from build123d import *

# Parameters (mm, degrees)
SKETCH1_W           = 20.32
SKETCH1_H           = 50.8
BOSS_EXTRUDE1_DEPTH = 19.05
CUT_EXTRUDE1_DEPTH  = 50.8
SKETCH5_W           = 3.175
SKETCH5_H           = 3.175
CUT_EXTRUDE2_DEPTH  = 50.8


with BuildPart() as part:
    # Sketch1 → Boss-Extrude1 (new body)
    with BuildSketch(Plane(origin=(0, 0, 0), x_dir=(1, 0, 0), z_dir=(0, 1, 0))):
        Rectangle(SKETCH1_W, SKETCH1_H)
    extrude(amount=BOSS_EXTRUDE1_DEPTH)

    # Sketch3 → Cut-Extrude1 (cut)
    with BuildSketch(Plane.XY.offset(25.4)):
        Polygon((-4.233333333, 3.81), (4.233333333, 3.81), (2.116666667, 1.905), (4.233333333, 0), (-4.233333333, 0), (-2.116666667, 1.905), align=None)
    extrude(amount=-CUT_EXTRUDE1_DEPTH, mode=Mode.SUBTRACT)

    # Sketch4 → Revolve1 (revolve)
    with BuildSketch(Plane.XZ.offset(-3.81)):
        with BuildLine():
            Line((0, 4.7413418), (0, 3.4713418))
            ThreePointArc((0, 3.4713418), (0.635, 4.1063418), (0, 4.7413418))
        make_face()
    revolve(axis=Axis((0, 3.81, -25.4), (0, 0, 1)))

    # Sketch5 → Cut-Extrude2 (cut)
    with BuildSketch(Plane.XY.offset(25.4)):
        with BuildLine():
            Line((-10.16, 6.35), (-10.16, 19.05))
            Line((-10.16, 19.05), (10.16, 19.05))
            Line((10.16, 19.05), (10.16, 6.35))
            ThreePointArc((10.16, 6.35), (0, 12.99479824), (-10.16, 6.35))
        make_face()
        with Locations((0, 7.9375)):
            Rectangle(SKETCH5_W, SKETCH5_H)
        with Locations((-5.08, 7.9375)):
            Rectangle(SKETCH5_W, SKETCH5_H)
        with Locations((5.08, 7.9375)):
            Rectangle(SKETCH5_W, SKETCH5_H)
    extrude(amount=-CUT_EXTRUDE2_DEPTH, mode=Mode.SUBTRACT)


solid = part.part
Can you work these out from the model? Positions are in its coordinate system, mm. A direction names the side the tool comes from. Coordinates: 2 decimals unless noted, no trailing zeros. Write each loop counter-clockwise with the first axis right and the second up, starting at its lowest first coordinate (ties: lowest second). Pieces come first, ordered by that corner, then holes.
Q1. Which directions (+Z, -Z, +X, -X, +Y, -Y) give clear straight access to the entire face, cutting with the end or side of a thin tool? Please do faces 4 (the face through (6.668, 8, 0)), 5 (the face through (0, 5, 25.4)), 6 (the face through (3.16, 0.966, 0.356)).
Results found:
face 4: +Z, -Z
face 5: +Z, +X, -X, +Y, -Y
face 6: +Z, -Z, -Y
Q2. Imagine slicing it at C-C, the plane y = 8.75. List the corners of the cut face in (x, z) for me.
Results found:
outline: (-8.73, -25.4) - (-6.67, -25.4) - (-6.67, 25.4) - (-8.73, 25.4) - close; (-3.49, -25.4) - (-1.59, -25.4) - (-1.59, 25.4) - (-3.49, 25.4) - close; (1.59, -25.4) - (3.49, -25.4) - (3.49, 25.4) - (1.59, 25.4) - close; (6.67, -25.4) - (8.73, -25.4) - (8.73, 25.4) - (6.67, 25.4) - close
Q3. Imagine slicing it at D-D, the plane y = 12. List the corners of the cut face in (x, z) for me, plus the area to 3 significant figures.
Results found:
outline: (-4.59, -25.4) - (4.59, -25.4) - (4.59, 25.4) - (-4.59, 25.4) - close
area: 466 mm2
Q4. Please list where these lines run through material, in increasing order: L1, parallel to X at y = 2, z = 9.5; L2, parallel to Y at x = -3.75, z = -16 (3 decimals); L3, parallel to Y at x = -1.5, z = -14.5 (3 decimals).
Results found:
L1: x = -10.16 to -2.22, 2.22 to 10.16
L2: y = 0.435 to 3.375, 3.81 to 6.35, 9.525 to 12.342
L3: y = 3.81 to 6.35, 9.525 to 12.893
Q5. Imagine slicing it at A-A, the plane z = 3. Count the separate pieces of the cut face and the enclosed holes in it, plus the area to 3 significant figures.
Results found:
separate pieces: 1
enclosed holes: 3
area: 172 mm2
Q6. For P1, Ø2.5, axis at y = 8, z = -9, coming from the -X side; P2, Ø5, axis at x = 5.5, z = 15, coming from the +Y side; P3, Ø2.5, axis at x = 5.5, z = -7, coming from the +Y side, each with a flat end and sliding along its axis, tell me the tip position at first contact or that it passes through.
Results found:
P1: stops at x = -9.98
P2: stops at y = 12.58
P3: stops at y = 12.15
Q7. If we mould it in two halves opening along X, with no side actions, what happens to faces 1 (the face through (-3.492, 8, 0)), 2 (the face through (7, 0, 0)), 3 (the face through (-10.16, 3, 0))? For each: +X half, -X half, draft (parallel to the pull), parting line (faces both ways), or undercut.
Results found:
face 1: undercut
face 2: draft
face 3: -X half
